Could you check a few things on this model? Use its own coordinates, in mm. Face numbers are marked on the shaded views. A direction names the side the tool comes from. Coordinates: 2 decimals unless noted, no trailing zeros. Loops run counter-clockwise (first coordinate to the right, second up) from the corner with the lowest first, then second, coordinate; pieces in that order, holes last. Notation, with made-up numbers: (-21, -11.75) - (-10, -11.75) arc R33 ccw to (-10, 23.25) - close; hole circle Ø3 at (41.5, 75). An arc over 180 degrees is marked (long way). One line per item, written item: value. Start each with the question number.
(1) If we mould it in two halves opening along X, with no side actions, what happens to the marked faces 3 and 4? For each: pulls with the +X half, pulls with the -X half, needs draft (parallel to the pull), parting line crosses it, or undercut.
(2) If I drill on line 1 along Y through (x, z) = (5.5, -0.25); line 2 along X through (y, z) = (0, 0.25); line 3 along X through (y, z) = (0.5, 2.25), over which ranges is the centre line in solid material (lowest first)? Write a range as from..to.
(3) If we section it at C-C on x = 57.5: Write out the boundary of the cut face in (y, z).
(4) I'm going to push flat-ended pins straight in: P1, Ø2, axis at y = 2, z = -4.5, coming from the -X side; P2, Ø5, axis at y = -2, z = -2.5, coming from the -X side; P3, Ø6, axis at x = 45.5, y = 1.5, coming from the -Z side. Where does each tip first touch, or does it pass through?
(5) If we section it at D-D on x = 5.5: Write out the boundary of the cut face in (y, z).
(6) On a 3-axis mill with a long thin cutter (end or side, diameter ignored), from which of +Z, -Z, +X, -X, +Y, -Y can I reach the whole of each face in a straight line? I mean the marked faces 1 and 2. Say none if no direction works.
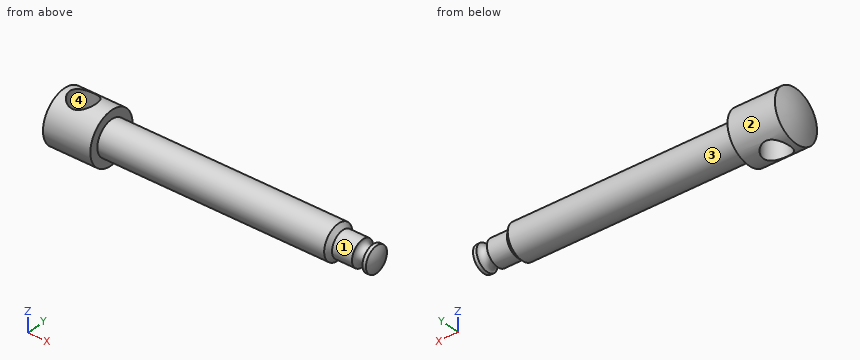
Autodesk Inventor part; units mm, degrees
ref_plane "Work Plane1" through (6.547, 0, 6) normal (0, 0, 1) x (1, 0, 0)
ref_plane "YZ Plane" through (0, 0, 0) normal (1, 0, 0) x (0, 1, 0)
ref_plane "XZ Plane" through (0, 0, 0) normal (0, 1, 0) x (-1, 0, 0)
sketch "Sketch1" plane through (0, 0, 0) normal (0, 0, 1) x (1, 0, 0)
  line L0 (0, 0) -> (74, 0)
  line L1 (0, 0) -> (17, 0)
  circle A0 centre (17, 0) radius 17
  line L2 (0, 0) -> (0, 12)
  line L3 (74, 0) -> (69, 0)
  circle A1 centre (69, 0) radius 5
  line L4 (74, 0) -> (74, 3)
  line L5 (74, 3) -> (65.2, 3)
  line L6 (65.2, 3) -> (65.2, 0)
  line L7 (65.2, 0) -> (74, 0)
  line L8 (74, 0) -> (74, 3)
  line L9 (74, 3) -> (69.8, 3)
  line L10 (69.8, 3) -> (69.8, 3)
  line L11 (69.8, 0) -> (74, 0)
  line L12 (74, 0) -> (74, 3)
  line L13 (74, 0) -> (69.8, 0)
  line L14 (69.8, 0) -> (69.8, 1.8)
  line L15 (71, 1.8) -> (74, 1.8)
  line L16 (74, 1.8) -> (74, 0)
  arc A2 (69.8, 3) -> (71, 1.8) centre (71, 3) ccw
  line L17 (71, 1.8) -> (71, 1.8)
  line L18 (72.2, 3) -> (72.2, 3)
  arc A3 (71, 1.8) -> (72.2, 3) centre (71, 3) ccw
  line L19 (65.2, 0) -> (12, 0)
  line L20 (12, 0) -> (12, 4)
  line L21 (12, 4) -> (65.2, 4)
  line L22 (65.2, 4) -> (65.2, 0)
  line L23 (12, 0) -> (0, 0)
  line L24 (0, 0) -> (0, 6)
  line L25 (0, 6) -> (12, 6)
  line L26 (12, 6) -> (12, 0)
  line L27 (12, 6) -> (5.5, 6)
  line L28 (5.5, 6) -> (5.5, 0)
  point P0 (72.2, 1.8)
  point P1 (1.094, 6)
  point P2 (73, 3)
  dimension "d0" = 74
  dimension "d1" = 17
  dimension "d2" = 12
  dimension "d3" = 5
  dimension "d4" = 3
  dimension "d5" = 8.8
  dimension "d6" = 4.2
  dimension "d7" = 1.8
  dimension "d8" = 1.2
  dimension "d9" = 1.2
  dimension "d10" = 1.2
  dimension "d11" = 53.2
  dimension "d12" = 4
  dimension "d13" = 6
  dimension "d14" = 6.5
revolve "Revolution1" add sketch "Sketch1" angle 360 about axis through (65.2, 0, 0) along (-1, 0, 0) contours A0 L25 L28 L0 | L28 L25 L26 L20 L0 | A0 L21 L22 A1 L0 | L0 L20 L21 A0 | A1 L22 L6 L0 | L6 L5 A2 L15 A1 L0 | A1 L15 A3 L5
chamfer "Chamfer1" distance 1 angle 45 1 edges at (65.2, -4, 0)
ref_plane "Work Plane1" through (6.547, 0, 6) normal (0, 0, 1) x (1, 0, 0)
sketch "Sketch2" plane through (6.547, 0, 6) normal (0, 0, 1) x (1, 0, 0)
  line L0 (5.453, 4) -> (5.453, -4)
  line L1 (5.453, 0) -> (-1.047, 0)
  circle A0 centre (-1.047, 0) radius 3.1
  point P0 (-6.547, 0)
  dimension "d19" = 6.5
  dimension "d20" = 6.2
extrude "Extrusion1" cut sketch "Sketch2" against normal through all
thread "Thread1"
properties part number "Menetesorsó"
Values:
1. face 3: needs draft
1. face 4: undercut
2. line 1: y = -5.99..-3.1, 3.1..5.99
2. line 2: x = 0..2.4, 8.6..73.99
2. line 3: x = 0.16..2.44, 8.56..70.02, 71.98..73.44
3. outline: circle Ø8 at (0, 0)
4. P1: stops at x = 0.46
4. P2: stops at x = 0.01
4. P3: stops at z = -4
5. outline: (-3.1, -5.14) - (-3.1, 5.14) arc R6 ccw to start; (3.1, -5.14) arc R6 ccw to (3.1, 5.14) - close
6. face 1: +X
6. face 2: +X, -X
